Source: CAD feature listing. Evaluate the final solid. Frame: model axes, mm. A direction names the side the tool comes from. Give positions to 0.01 mm unless a question says otherwise; leave off trailing zeros. Order: outer loops, then holes, each group sorted by start corner. A loop starts at its lowest first (then second) coordinate and runs counter-clockwise, first axis right, second up.
from build123d import *

# Parameters (mm, degrees)
EXTRUDE_1_DEPTH      = 50
SHELL_2_T            = -3
SKETCH_13_R          = 4
CUT_EXTRUDE_1_DEPTH  = 250
SKETCH_18_R          = 25
EXTRUDE_4_DEPTH      = 2
SKETCH_19_R          = 9.153493009
CUT_EXTRUDE_10_DEPTH = 65.852487738
SKETCH_16_R          = 25
EXTRUDE_3_DEPTH      = 2
SKETCH_17_R          = 23
CUT_EXTRUDE_9_DEPTH  = 65.852487738


with BuildPart() as part:
    # 草图1 → 凸台-拉伸1 (new body)
    with BuildSketch(Plane.XY):
        with BuildLine():
            Line((-22.5, -10.897247359), (-22.5, -30.897247359))
            Line((-22.5, -30.897247359), (22.5, -30.897247359))
            Line((22.5, -30.897247359), (22.5, -10.897247359))
            ThreePointArc((22.5, -10.897247359), (0, 25), (-22.5, -10.897247359))
        make_face()
    extrude(amount=EXTRUDE_1_DEPTH)

    # 抽壳2
    shell_2_openings = [part.faces().sort_by_distance(p)[0] for p in [
        (0, -4.655282496, 0),
        (0, -30.897247359, 25),
    ]]
    offset(amount=SHELL_2_T, openings=shell_2_openings, kind=Kind.INTERSECTION)

    # 草图13 → 切除-拉伸1 (cut, symmetric)
    with BuildSketch(Plane(origin=(0, 0, 0), x_dir=(0, 0, -1), z_dir=(1, 0, 0))):
        with Locations(Location((-7, -24, 0), (0, 0, 180))):
            Circle(SKETCH_13_R)
        with BuildLine():
            Line((-40, 25.208572912), (-1.432281326, -22.471249301))
            ThreePointArc((-1.432281326, -22.471249301), (-1.063231061, -27.254219062), (-4.184343468, -30.897247359))
            Line((-4.184343468, -30.897247359), (0, -30.897247359))
            Line((0, -30.897247359), (0, 25.208572912))
            Line((0, 25.208572912), (-40, 25.208572912))
        make_face()
    extrude(amount=CUT_EXTRUDE_1_DEPTH, both=True, mode=Mode.SUBTRACT)

    # 草图18 → 凸台-拉伸4 (add)
    with BuildSketch(Plane.XY.offset(50)):
        with Locations(Location((0, 0, 0), (0, 0, 205.841932763))):
            Circle(SKETCH_18_R)
    extrude(amount=EXTRUDE_4_DEPTH)

    # 圆角3: read off the stored shape, not the designer's step
    # 圆角3 outline → 圆角3 (revolve, cut)
    with BuildSketch(Plane.XZ):
        with BuildLine():
            ThreePointArc((23, 52), (24.414213562, 51.414213562), (25, 50))
            Line((25, 50), (25, 52))
            Line((25, 52), (23, 52))
        make_face()
    revolve(axis=Axis((0, 0, 0), (0, 0, 1)), mode=Mode.SUBTRACT)

    # 草图19 → 切除-拉伸10 (cut, through all)
    with BuildSketch(Plane.XY.offset(52)):
        Circle(SKETCH_19_R)
    extrude(amount=-CUT_EXTRUDE_10_DEPTH, mode=Mode.SUBTRACT)

    # 草图16 → 凸台-拉伸3 (add)
    with BuildSketch(Plane.XY.offset(50)):
        with Locations(Location((0, 0, 0), (0, 0, 205.841932763))):
            Circle(SKETCH_16_R)
    extrude(amount=EXTRUDE_3_DEPTH)

    # 圆角2: read off the stored shape, not the designer's step
    # 圆角2 outline → 圆角2 (revolve, cut)
    with BuildSketch(Plane.XZ):
        with BuildLine():
            ThreePointArc((23, 52), (24.414213562, 51.414213562), (25, 50))
            Line((25, 50), (25, 52))
            Line((25, 52), (23, 52))
        make_face()
    revolve(axis=Axis((0, 0, 0), (0, 0, 1)), mode=Mode.SUBTRACT)

    # 草图17 → 切除-拉伸9 (cut, through all)
    with BuildSketch(Plane.XY.offset(52)):
        Circle(SKETCH_17_R)
    extrude(amount=-CUT_EXTRUDE_9_DEPTH, mode=Mode.SUBTRACT)


solid = part.part
(1) Access query for faces 1 (the flat face through (19.5, -22, 24)), 2 (the flat face through (22.5, -21, 25)), 3 (the cylindrical face through (20.979, -27.966, 6.479)). Directions: +Z, -Z, +X, -X, +Y, -Y. A direction counts if a zero-diameter tool reaches every point of the face in a straight line with its end or side. Return the directions, or none.
(2) Section A-A, the plane z = 7. Return loops of the section in (x, y).
(3) Pin query (flat end, axial travel): pin 1 Ø8 at (x, z) = (-15, 42.5) entering from -Y; pin 2 Ø9.5 at (x, y) = (-1, -23) entering from -Z; pin 3 Ø3 at (y, z) = (-17, 31) entering from -X; pin 4 Ø12 at (x, z) = (-13.5, 43) entering from -Y. Return the tip coordinate at first contact, or that it passes through.
(4) Section B-B, the plane y = 0. Return loops of the section in (x, z), plus the area to 3 significant figures.
(5) Line query: line 1 along X through (y, z) = (-17.5, 21); line 2 along X through (y, z) = (0, 29); line 3 along Y through (x, z) = (-20.25, 7). Output: solid intervals per line, ascending.
(6) Section C-C, the plane y = -24. Count the separate pieces of the cut face and the enclosed holes in it, plus the area to 3 significant figures.
(7) Draft query along X for faces 4 (the flat face through (0, -26, 47)), 5 (the flat face through (-0.3, -25.2, 50)), 6 (the flat face through (-22.5, -21, 25)). Return one class per face: +X half, -X half, draft (parallel to the pull), parting line (faces both ways), or undercut.
Checks:
1. face 1: -Z, -Y
1. face 2: +Z, -Z, +X, -Y
1. face 3: +X, -X
2. outline: (-22.5, -30.9) - (-19.5, -30.9) - (-19.5, -28) - (-22.5, -28) - close; (-22.5, -20) - (-19.5, -20) - (-19.5, -15.59) - (-22.5, -15.59) - close; (19.5, -30.9) - (22.5, -30.9) - (22.5, -28) - (19.5, -28) - close; (19.5, -20) - (22.5, -20) - (22.5, -15.59) - (19.5, -15.59) - close
3. pin 1: stops at y = 12.96
3. pin 2: stops at z = 47
3. pin 3: stops at x = -22.5
3. pin 4: stops at y = -30.9
4. outline: (-25, 19.61) - (-23, 19.61) - (-23, 52) arc R2 ccw to (-25, 50) - close; (23, 19.61) - (25, 19.61) - (25, 50) arc R2 ccw to (23, 52) - close
4. area: 128 mm2
5. line 1: x = -22.5 to -19.5, 19.5 to 22.5
5. line 2: x = -25 to -23, 23 to 25
5. line 3: y = -30.9 to -28, -20 to -15.59
6. separate pieces: 3
6. enclosed holes: 0
6. area: 383 mm2
7. face 4: undercut
7. face 5: draft
7. face 6: -X half
